```python
from build123d import *

# Parameters (mm, degrees)
F0_W        = 83.6402177811
F0_H        = 18.8771318644
F1_DEPTH    = 12.7
F2_DEPTH    = 6.35
F3_T4_DEPTH = 183.094881238
F4_T4_DEPTH = 183.094881238
F5_R        = 7.62
F6_R        = 7.62
F7_W        = 2.0920878742
F7_H        = 68.6837211251


# Not quite as in the source:
# - a fillet or chamfer that OpenCascade refuses, or shapes differently, is made with other operations: its cross-section is extruded or revolved along the edge and cut away or added


with BuildPart() as f1:
    # F0 (on Right) → F1 (new body, symmetric)
    with BuildSketch(Plane.YZ):
        with BuildLine():
            ThreePointArc((-74.9276950955, 9.4385659322), (-60.8756748212, -4.3877247968), (-41.8201088905, -9.4385659322))
            Line((-41.8201088905, -9.4385659322), (-74.9276950955, 9.4385659322))
        make_face()
        with BuildLine():
            Line((74.9276950955, 9.4385659322), (41.8201088905, -9.4385659322))
            ThreePointArc((41.8201088905, -9.4385659322), (60.8756748212, -4.3877247968), (74.9276950955, 9.4385659322))
        make_face()
        Polygon((74.9276950955, 9.4385659322), (41.8201088905, 9.4385659322), (41.8201088905, -9.4385659322), align=None)
        Rectangle(F0_W, F0_H)
        Polygon((-41.8201088905, -9.4385659322), (-41.8201088905, 9.4385659322), (-74.9276950955, 9.4385659322), align=None)
    extrude(amount=F1_DEPTH, both=True)

    # F0 (on Right) → F2 (join, symmetric)
    with BuildSketch(Plane.YZ):
        Polygon((41.8201088905, -9.4385659322), (-41.8201088905, -9.4385659322), (-30.2034132183, -21.926516667), (54.0176406503, -21.3456805795), align=None)
    extrude(amount=F2_DEPTH, both=True)

    # F3: chamfer of 19.05 x 6.35 on 1 edges, made by hand


with BuildPart() as f3_tool2:
    # F3_s3 → F3_t4 (new body)
    with BuildSketch(Plane(origin=(0, -79.7879238623, -0.5502627122), x_dir=(1, 0, 0), z_dir=(0, 0.9999762195, 0.0068964024))):
        Polygon((-6.35, 2.6677003539), (0, 21.7177003539), (-6.35, 21.7177003539), align=None)
    extrude(amount=F3_T4_DEPTH)

    split(bisect_by=Plane.XY.offset(-9.4385659322), keep=Keep.BOTTOM)


with BuildPart() as f1_1:
    add(f1.part)

    # F3_t1: cut F3_tool2
    add(f3_tool2.part, mode=Mode.SUBTRACT)

    # F4: chamfer of 6.35 x 19.05 on 1 edges, made by hand


with BuildPart() as f4_tool2:
    # F4_s3 → F4_t4 (new body)
    with BuildSketch(Plane(origin=(0, -79.7879238623, -0.5502627122), x_dir=(1, 0, 0), z_dir=(0, 0.9999762195, 0.0068964024))):
        Polygon((6.35, 2.6677003539), (0, 21.7177003539), (6.35, 21.7177003539), align=None)
    extrude(amount=F4_T4_DEPTH)

    split(bisect_by=Plane.XY.offset(-9.4385659322), keep=Keep.BOTTOM)


with BuildPart() as f1_2:
    add(f1_1.part)

    # F4_t1: cut F4_tool2
    add(f4_tool2.part, mode=Mode.SUBTRACT)

    # F5
    f5_edges = [f1_2.edges().sort_by_distance(p)[0] for p in [
        (-12.7, 60.875675, -4.387725),
        (-12.7, 0, -9.438566),
        (-12.7, -60.875675, -4.387725),
    ]]
    fillet(f5_edges, radius=F5_R)

    # F6
    f6_edges = [f1_2.edges().sort_by_distance(p)[0] for p in [
        (12.7, -60.875675, -4.387725),
        (12.7, 0, -9.438566),
        (12.7, 60.875675, -4.387725),
    ]]
    fillet(f6_edges, radius=F6_R)

    # F7 (on Right) → F8 (revolve)
    with BuildSketch(Plane.YZ):
        with Locations((1.0460439371, 34.3418605626)):
            Rectangle(F7_W, F7_H)
    revolve(axis=Axis((0, 0, 34.3418605626), (0, 0, 1)))


solid = f1_2.part
```
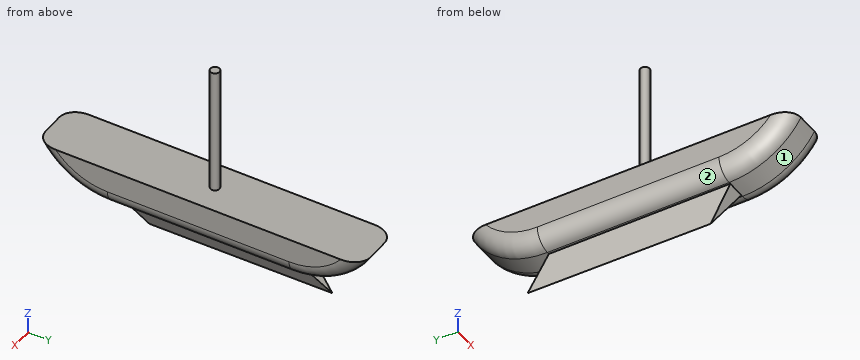
Can you work these out from the model? Positions are in its coordinate system, mm. Face numbers are marked on the shaded views. Coordinates: 2 decimals unless noted, no trailing zeros. Loops run counter-clockwise (first coordinate to the right, second up) from the corner with the lowest first, then second, coordinate; pieces in that order, holes last.
Item 1: Suppose I cut it at B-B (z = 15.5). Please give me the cut outline in (x, y), then the cut area to 3 significant figures.
Answers below:
outline: circle Ø4.18 at (0, 0)
area: 13.8 mm2
Item 2: I'm going to push flat-ended pins straight in: pin 1 (8 mm diameter, centred on x = 0, y = -21, fed in from +Z); pin 2 (2 mm diameter, centred on x = -7, y = -6, fed in from -Z). Where does each tip first touch, or does it pass through?
Answers below:
pin 1: stops at z = 9.44
pin 2: stops at z = -9.38
Item 3: Please list where these lines run through material, in increasing order: L1, parallel to Z at x = 1.25, y = -61.5; L2, parallel to Z at x = -5.5, y = -7; L3, parallel to Y at x = -8.5, z = 5.
Answers below:
L1: z = -4.02 to 9.44
L2: z = -9.43 to 9.44
L3: y = -70.82 to 70.82
Item 4: Suppose I cut it at A-A (y = 7). Please give me the cut outline in (x, z), then the cut area to 3 significant figures.
Answers below:
outline: (-12.7, -1.82) arc R7.62 ccw to (-5.08, -9.44) - (-4.08, -9.44) - (0, -21.67) - (4.08, -9.44) - (5.08, -9.44) arc R7.62 ccw to (12.7, -1.82) - (12.7, 9.44) - (-12.7, 9.44) - close
area: 504 mm2
Item 5: Suppose I cut it at C-C (y = -24). Please give me the cut outline in (x, z).
Answers below:
outline: (-12.7, -1.82) arc R7.62 ccw to (-5.08, -9.44) - (-4.15, -9.44) - (0, -21.88) - (4.15, -9.44) - (5.08, -9.44) arc R7.62 ccw to (12.7, -1.82) - (12.7, 9.44) - (-12.7, 9.44) - close
Item 6: If we mould it in two halves opening along Y, with no side actions, what happens to the marked faces 1 and 2? For each: released by +Y, released by -Y, zero draft, split by the parting line, or undercut.
Answers below:
face 1: released by -Y
face 2: zero draft
